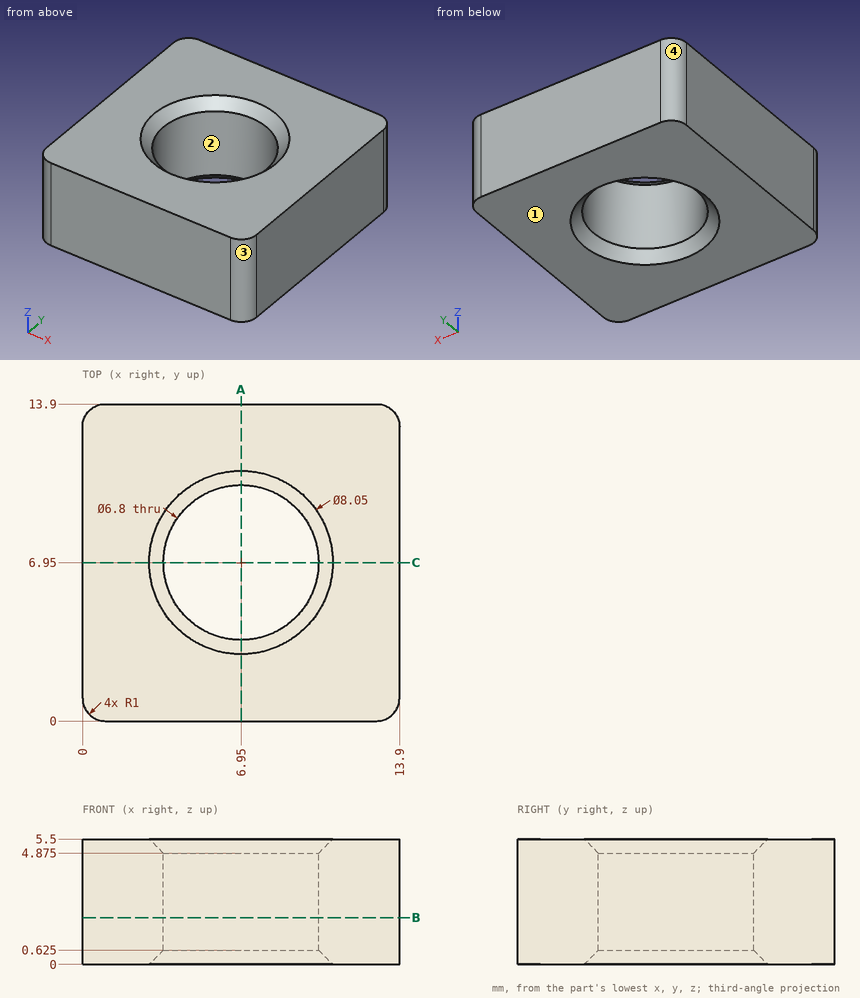
Input: dimensioned drawing with shaded views. Units: mm. Origin: part minimum x, y, z. Coordinates: 2 decimals unless noted, no trailing zeros. Order: outer loops, then holes, each group sorted by start corner. A loop starts at its lowest first (then second) coordinate and runs counter-clockwise, first axis right, second up.
(1) Section query B-B (z = 2.05). Return the cut outline in (x, y).
(2) Material intervals for probe 1 along X at (y, z) = (6.95, 2.35); probe 2 along X at (y, z) = (5, 4.5), sorted ascending.
(3) Section query A-A (x = 6.95). Return the cut outline in (y, z) (3 decimals), plus the area to 3 significant figures.
(4) Draft query along X for the marked faces 1, 2, 3 and 4. Return one class per face: pulls with the +X half, pulls with the -X half, needs draft (parallel to the pull), parting line crosses it, or undercut.
Solution:
1. outline: (0, 1) arc R1 ccw to (1, 0) - (12.9, 0) arc R1 ccw to (13.9, 1) - (13.9, 12.9) arc R1 ccw to (12.9, 13.9) - (1, 13.9) arc R1 ccw to (0, 12.9) - close; hole circle Ø6.8 at (6.95, 6.95)
2. probe 1: x = 0 to 3.55, 10.35 to 13.9
2. probe 2: x = 0 to 4.16, 9.74 to 13.9
3. outline: (0, 0) - (2.925, 0) - (3.55, 0.625) - (3.55, 4.875) - (2.925, 5.5) - (0, 5.5) - close; (10.35, 0.625) - (10.975, 0) - (13.9, 0) - (13.9, 5.5) - (10.975, 5.5) - (10.35, 4.875) - close
3. area: 38.3 mm2
4. face 1: needs draft
4. face 2: undercut
4. face 3: pulls with the +X half
4. face 4: pulls with the -X half
